Autodesk Inventor part; units mm, degrees
ref_plane "YZ Plane" through (0, 0, 0) normal (1, 0, 0) x (0, 1, 0)
ref_plane "XZ Plane" through (0, 0, 0) normal (0, 1, 0) x (-1, 0, 0)
ref_plane "XY Plane" through (0, 0, 0) normal (0, 0, 1) x (1, 0, 0)
sketch "草圖1" plane through (0, 0, 0) normal (0, 1, 0) x (-1, 0, 0)
  line L0 (0, 80) -> (9, 80)
  line L1 (9, -80) -> (0, -80)
  line L2 (0, -80) -> (0, 80)
  line L3 (7, 4.5) -> (2, 4.5)
  line L4 (2, 4.5) -> (2, -4.5)
  line L5 (2, -4.5) -> (7, -4.5)
  line L6 (9, 80) -> (9, 90)
  line L7 (9, 90) -> (-3, 90)
  line L8 (-8, 85) -> (-8, 85)
  line L9 (-3, 80) -> (0, 80)
  arc A0 (-8, 85) -> (-3, 80) centre (-3, 85) ccw
  arc A1 (-3, 90) -> (-8, 85) centre (-3, 85) ccw
  circle A2 centre (-3, 85) radius 2.5
  line L10 (9, 0) -> (0, 0)
  line L11 (9, -80) -> (9, -90)
  line L12 (9, -90) -> (-3, -90)
  line L13 (-3, -80) -> (0, -80)
  arc A3 (-3, -80) -> (-8, -85) centre (-3, -85) ccw
  arc A4 (-8, -85) -> (-3, -90) centre (-3, -85) ccw
  circle A5 centre (-3, -85) radius 2.5
  line L14 (9, 80) -> (9, 4.6)
  line L15 (9, -4.6) -> (9, -80)
  line L16 (7, -4.5) -> (7, -4.2)
  line L17 (7, -4.2) -> (9, -4.6)
  line L18 (7, 4.5) -> (7, 4.2)
  line L19 (7, 4.2) -> (9, 4.6)
  line L20 (9, 90) -> (0, 90)
  line L21 (0, 90) -> (0, 100)
  line L22 (0, 100) -> (9, 100)
  line L23 (9, 100) -> (9, 90)
  line L24 (9, -90) -> (0, -90)
  line L25 (0, -90) -> (0, -100)
  line L26 (0, -100) -> (9, -100)
  line L27 (9, -100) -> (9, -90)
  line L28 (2, 97) -> (7, 97)
  line L29 (7, 97) -> (7, 88)
  line L30 (7, 88) -> (2, 88)
  line L31 (2, 88) -> (2, 97)
  line L32 (7, -97) -> (2, -97)
  line L33 (2, -97) -> (2, -88)
  line L34 (2, -88) -> (7, -88)
  line L35 (7, -88) -> (7, -97)
  point P0 (4.5, 4.5)
  point P1 (4.5, 80)
  point P2 (-8, 90)
  point P3 (-8, -90)
  point P4 (2, 0)
  point P5 (4.5, 97)
  point P6 (4.5, 100)
  point P7 (4.5, -97)
  point P8 (4.5, -100)
  dimension "d0" = 160
  dimension "d1" = 9
  dimension "d3" = 5
  dimension "d4" = 10
  dimension "d5" = 17
  dimension "d6" = 5
  dimension "d7" = 5
  dimension "d8" = 5
  dimension "d13" = 9
  dimension "d14" = 0.3
  dimension "d15" = 0.3
  dimension "d17" = 0
  dimension "d18" = 5
  dimension "d21" = 17
  dimension "d22" = 10
  dimension "d23" = 9
  dimension "d24" = 9
  dimension "d25" = 10
  dimension "d26" = 9
  dimension "d27" = 5
  dimension "d28" = 3
  dimension "d29" = 9
  dimension "d30" = 5
  dimension "d31" = 3
  dimension "d32" = 75.4
  dimension "d33" = 75.4
extrude "擠出1" add sketch "草圖1" along normal blind 3 contours L9 A0 A1 L7 L31 L30 L29 L6 L0 | L0 L14 L19 L18 L3 L4 L10 L2 | L10 L4 L5 L16 L17 L15 L1 L2 | L7 L29 L28 L31 L21 L22 L23 | L1 L11 L12 L35 L34 L33 A4 A3 L13 | L27 L26 L25 L12 L33 L32 L35
properties part number "Lower_Bar" material "MDF Medium Density Fiberboard"
Work out the finished part from the listing and answer in its coordinate system (mm). Round coordinates to 2 decimals unless told otherwise and drop trailing zeros. Loops run counter-clockwise (first coordinate to the right, second up) from the corner with the lowest first, then second, coordinate; pieces in that order, holes last. Notation, with made-up numbers: M 87,36 L 145,36 A21 cw 145,43 Z; hole C 3,88 d3. An arc over 180 degrees is marked long. One line per question, with ' | ' between items.
Q1. The mould has two halves that part along X. Classify faces 1 (the cylindrical face through (3.33, 1.48, 82.52)), 2 (the flat face through (-4, 3, -21)), 3 (the cylindrical face through (8, 1, -85)): +X half, -X half, draft (parallel to the pull), parting line (faces both ways), or undercut.
Conclusion:
face 1: undercut | face 2: draft | face 3: +X half
Q2. Find section B-B, the plane z = -60. Give the vertices of the cut face in (x, y).
Conclusion:
outline: M -9,0 L 0,0 L 0,3 L -9,3 Z
Q3. Each of these flat-tipped pins is pushed along its axis until it touches: pin 1 Ø0.9 at (x, y) = (1, 1) entering from +Z; pin 2 Ø1.5 at (x, y) = (2, 1.5) entering from -Z. Where does it stop, or does it pass through?
Conclusion:
pin 1: stops at z = 90 | pin 2: stops at z = -90
Q4. Consider line 1 along Z through (x, y) = (3, 1.15); line 2 along Z through (x, y) = (-6.75, 1.7); line 3 along X through (y, z) = (1.65, 39.5). Determine where each line is inside the solid, lowest interval first. Write a range as from..to.
Conclusion:
line 1: z = -90..-87.5, -82.5..-80, 80..82.5, 87.5..90 | line 2: z = -100..-97, -88..-4.5, 4.5..88, 97..100 | line 3: x = -9..0
Q5. Find section A-A, the plane z = 85. Give the vertices of the cut face in (x, y), then the cut area to 3 significant figures.
Conclusion:
outline: M -9,0 L 0.5,0 L 0.5,3 L -9,3 Z; M 5.5,0 L 8,0 L 8,3 L 5.5,3 Z | area: 36.0 mm2
